from build123d import *

# Parameters (mm, degrees)
F0_W     = 914.4
F0_H     = 609.6
F1_DEPTH = 889
F2_W     = 63.5
F2_H     = 76.2
F3_DEPTH = 914.4
F4_W     = 397.184085
F4_H     = 642.411709
F4_W_2   = 404.053162
F5_DEPTH = 25.4


with BuildPart() as f1:
    # F0 (on Top) → F1 (new body)
    with BuildSketch(Plane.XY):
        Rectangle(F0_W, F0_H)
    extrude(amount=F1_DEPTH)

    # F2 (on face) → F3 (cut)
    with BuildSketch(Plane(origin=(-457.2, 0, 0), x_dir=(0, -1, 0), z_dir=(-1, 0, 0))):
        with Locations((-273.05, 38.1)):
            Rectangle(F2_W, F2_H)
    extrude(amount=-F3_DEPTH, mode=Mode.SUBTRACT)

    # F4 (on face) → F5 (cut)
    with BuildSketch(Plane(origin=(0, 304.8, 0), x_dir=(-1, 0, 0), z_dir=(0, 1, 0))):
        with Locations((-204.942043, 479.41935)):
            Rectangle(F4_W, F4_H)
        with Locations((208.376581, 479.41935)):
            Rectangle(F4_W_2, F4_H)
    extrude(amount=-F5_DEPTH, mode=Mode.SUBTRACT)


solid = f1.part
The listing builds one solid part. Answer for the finished solid, in the listing's coordinates (mm). A direction names the side the tool comes from. Round coordinates to 2 decimals unless told otherwise and drop trailing zeros. Write each loop counter-clockwise with the first axis right and the second up, starting at its lowest first coordinate (ties: lowest second). Pieces come first, ordered by that corner, then holes. Notation, with made-up numbers: (-28, 46.5) - (-1, 46.5) arc R12 ccw to (-1, 66.5) - close; hole circle Ø2 at (-6, 42). An arc over 180 degrees is marked (long way). Use a Markdown table: item, result. Add a question column.
1. Consider line 1 (Y direction, x = -70.5, z = 716); line 2 (Z direction, x = -131.5, y = 275.5). Determine where each line is inside the solid, lowest interval first.
2. Flat-ended cylindrical pins translate along their axes: P1, Ø7.5, axis at x = -187.5, y = 298, coming from the -Z side; P2, Ø1, axis at x = 83.5, y = -235.5, coming from the -Z side; P3, Ø3, axis at x = -276.5, z = 388.5, coming from the +Y side. Find the tip coordinate at first contact, or state that the pin passes through.
3. For a pull along Z with two mould halves and no side action, classify faces 1 (the face through (403.534, 292, 475)), 2 (the face through (-6, 273, 76.2)), 3 (the face through (-457.2, -4, 438)), 4 (the face through (6.35, 292, 475)) as +Z half, -Z half, draft (parallel to the pull), parting line (faces both ways), or undercut.
4. The part is cut by section A-A (x = 328.5). Write down the section's boundary in (y, z), and give its area (3 significant figures).
5. A tool of negligible diameter and unlimited length cuts with its end or side. For faces 5 (the face through (-206, 279.4, 484)), 6 (the face through (-6, 241.3, 38)), 7 (the face through (-2, 304.8, 481)), from which of +Z, -Z, +X, -X, +Y, -Y can it reach the whole face along a straight path? Write none if from no direction.
6. The part is cut by section B-B (z = 561). Write down the section's boundary in (x, y).
Reported:
| question | item | result |
|---|---|---|
| 1 | line 1 | -304.8 to 279.4 |
| 1 | line 2 | 76.2 to 889 |
| 2 | P1 | z = 76.2 |
| 2 | P2 | z = 0 |
| 2 | P3 | y = 279.4 |
| 3 | face 1 | undercut |
| 3 | face 2 | -Z half |
| 3 | face 3 | draft |
| 3 | face 4 | undercut |
| 4 | outline | (-304.8, 0) - (241.3, 0) - (241.3, 76.2) - (304.8, 76.2) - (304.8, 158.21) - (279.4, 158.21) - (279.4, 800.63) - (304.8, 800.63) - (304.8, 889) - (-304.8, 889) - close |
| 4 | area | 521,000 mm^2 |
| 5 | face 5 | +Y |
| 5 | face 6 | -Z, +X, -X, +Y |
| 5 | face 7 | +Z, -Z, +X, -X, +Y |
| 6 | outline | (-457.2, -304.8) - (457.2, -304.8) - (457.2, 304.8) - (403.53, 304.8) - (403.53, 279.4) - (6.35, 279.4) - (6.35, 304.8) - (-6.35, 304.8) - (-6.35, 279.4) - (-410.4, 279.4) - (-410.4, 304.8) - (-457.2, 304.8) - close |
